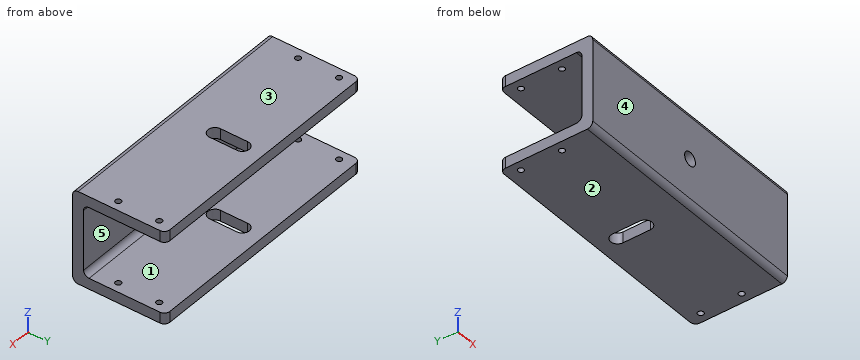
from build123d import *

# Parameters (mm, degrees)
SKETCH_1_W          = 92
SKETCH_1_H          = 30
SKETCH_1_R          = 1.05
EXTRUDE_1_DEPTH     = 4
SKETCH_4_W          = 92
SKETCH_4_H          = 30
EXTRUDE_4_DEPTH     = 4
SKETCH_5_W          = 92
SKETCH_5_H          = 34
SKETCH_5_R          = 1.05
EXTRUDE_5_DEPTH     = 4
FILLET_4_R          = 2
CUT_EXTRUDE_1_DEPTH = 45
SKETCH_8_R          = 2.55
CUT_EXTRUDE_2_DEPTH = 5


with BuildPart() as part:
    # 草图1 → 凸台-拉伸1 (new body)
    with BuildSketch(Plane.XY):
        with Locations((46, -15)):
            Rectangle(SKETCH_1_W, SKETCH_1_H)
        with Locations((3.5, -5)):
            Circle(SKETCH_1_R, mode=Mode.SUBTRACT)
        with Locations((3.5, -20)):
            Circle(SKETCH_1_R, mode=Mode.SUBTRACT)
        with Locations((88.5, -5)):
            Circle(SKETCH_1_R, mode=Mode.SUBTRACT)
        with Locations((88.5, -20)):
            Circle(SKETCH_1_R, mode=Mode.SUBTRACT)
        with BuildLine():
            Line((43.45, -17.5), (43.45, -7.5))
            ThreePointArc((43.45, -7.5), (46, -4.95), (48.55, -7.5))
            Line((48.55, -7.5), (48.55, -17.5))
            ThreePointArc((48.55, -17.5), (46, -20.05), (43.45, -17.5))
        make_face(mode=Mode.SUBTRACT)
    extrude(amount=EXTRUDE_1_DEPTH)

    # 草图4 → 凸台-拉伸4 (add)
    with BuildSketch(Plane(origin=(0, -30, 0), x_dir=(-1, 0, 0), z_dir=(0, -1, 0))):
        with Locations((-46, -15)):
            Rectangle(SKETCH_4_W, SKETCH_4_H)
    extrude(amount=EXTRUDE_4_DEPTH)

    # 草图5 → 凸台-拉伸5 (add)
    with BuildSketch(Plane.XY.offset(30)):
        with Locations((46, -17)):
            Rectangle(SKETCH_5_W, SKETCH_5_H)
        with Locations((3.5, -5)):
            Circle(SKETCH_5_R, mode=Mode.SUBTRACT)
        with Locations((3.5, -20)):
            Circle(SKETCH_5_R, mode=Mode.SUBTRACT)
        with Locations((88.5, -20)):
            Circle(SKETCH_5_R, mode=Mode.SUBTRACT)
        with Locations((88.5, -5)):
            Circle(SKETCH_5_R, mode=Mode.SUBTRACT)
    extrude(amount=EXTRUDE_5_DEPTH)

    # 圆角4
    fillet_4_edges = [part.edges().sort_by_distance(p)[0] for p in [
        (46, -30, 30),
        (46, -34, 0),
        (46, -34, 34),
        (0, 0, 32),
        (92, 0, 32),
        (0, 0, 2),
        (92, 0, 2),
        (46, -30, 4),
    ]]
    fillet(fillet_4_edges, radius=FILLET_4_R)

    # 草图7 → 切除-拉伸1 (cut)
    with BuildSketch(Plane(origin=(0, 0, 0), x_dir=(-1, 0, 0), z_dir=(0, 0, -1))):
        with BuildLine():
            Line((-48.55, -17.5), (-48.55, -7.5))
            ThreePointArc((-48.55, -7.5), (-46, -4.95), (-43.45, -7.5))
            Line((-43.45, -7.5), (-43.45, -17.5))
            ThreePointArc((-43.45, -17.5), (-46, -20.05), (-48.55, -17.5))
        make_face()
    extrude(amount=-CUT_EXTRUDE_1_DEPTH, mode=Mode.SUBTRACT)

    # 草图8 → 切除-拉伸2 (cut)
    with BuildSketch(Plane(origin=(0, -34, 0), x_dir=(-1, 0, 0), z_dir=(0, -1, 0))):
        with Locations(Location((-46, -16.5, 0), (0, 0, 90))):
            Circle(SKETCH_8_R)
    extrude(amount=-CUT_EXTRUDE_2_DEPTH, mode=Mode.SUBTRACT)


solid = part.part
For this review, take the finished solid that the model builds, in its own axes (mm). Face numbers are marked on the shaded views. A direction names the side the tool comes from. Round coordinates to 2 decimals unless told otherwise and drop trailing zeros. Loops run counter-clockwise (first coordinate to the right, second up) from the corner with the lowest first, then second, coordinate; pieces in that order, holes last. Notation, with made-up numbers: (74.5, -39.75) - (119.5, -39.75) arc R7 ccw to (119.5, -26.75) - close; hole circle Ø11 at (53.5, 79). An arc over 180 degrees is marked (long way). Answer as CSV lines item,"result".
(1) Consider section A-A on x = 3.5. Give the boundary of the cut face in (y, z).
Checked values:
outline,"(-34, 2) arc R2 ccw to (-32, 0) - (-21.05, 0) - (-21.05, 4) - (-28, 4) arc R2 cw to (-30, 6) - (-30, 28) arc R2 cw to (-28, 30) - (-21.05, 30) - (-21.05, 34) - (-32, 34) arc R2 ccw to (-34, 32) - close; (-18.95, 0) - (-6.05, 0) - (-6.05, 4) - (-18.95, 4) - close; (-18.95, 30) - (-6.05, 30) - (-6.05, 34) - (-18.95, 34) - close; (-3.95, 0) - (0, 0) - (0, 4) - (-3.95, 4) - close; (-3.95, 30) - (0, 30) - (0, 34) - (-3.95, 34) - close"
(2) Wall thickness on line 1 (Z direction, x = 12, y = -22.5); line 2 (Y direction, x = 88.5, z = 2); line 3 (X direction, y = -32.85, z = 16.5): over which ranges is each line inside the solid? List them lowest first.
Checked values:
line 1,"z = 0 to 4, 30 to 34"
line 2,"y = -34 to -21.05, -18.95 to -6.05, -3.95 to 0"
line 3,"x = 0 to 43.45, 48.55 to 92"
(3) Consider section D-D on z = 16.5. Give the boundary of the cut face in (x, y), then the cut area to 3 significant figures.
Checked values:
outline,"(0, -34) - (43.45, -34) - (43.45, -30) - (0, -30) - close; (48.55, -34) - (92, -34) - (92, -30) - (48.55, -30) - close"
area,"348 mm2"
(4) Consider section C-C on y = -24.5. Give the boundary of the cut face in (x, z).
Checked values:
outline,"(0, 0) - (92, 0) - (92, 4) - (0, 4) - close; (0, 30) - (92, 30) - (92, 34) - (0, 34) - close"
(5) Tool access review of the marked faces 4 and 5: name each direction out of +Z, -Z, +X, -X, +Y, -Y from which nothing blocks a thin tool from reaching the whole face with its end or side.
Checked values:
face 4,"+Z, -Z, +X, -X, -Y"
face 5,"+X, -X, +Y"
(6) Insertion check: P1, Ø10, axis at x = 49, z = 19, coming from the +Y side. The pin has a flat end and moves straight along its axis. Give the tip position at first contact, or say it passes through.
Checked values:
P1,"stops at y = -30"
(7) Mouldability with a two-part tool opening along Z and no side actions: class the marked faces 1, 2 and 3 as +Z half, -Z half, draft (parallel to the pull), parting line (faces both ways), or undercut.
Checked values:
face 1,"undercut"
face 2,"-Z half"
face 3,"+Z half"
(8) Consider section B-B on y = -11. Give the boundary of the cut face in (x, z), then the cut area to 3 significant figures.
Checked values:
outline,"(0, 0) - (43.45, 0) - (43.45, 4) - (0, 4) - close; (0, 30) - (43.45, 30) - (43.45, 34) - (0, 34) - close; (48.55, 0) - (92, 0) - (92, 4) - (48.55, 4) - close; (48.55, 30) - (92, 30) - (92, 34) - (48.55, 34) - close"
area,"695 mm2"
